The listing builds one solid part. Answer for the finished solid, in the listing's coordinates (mm). A direction names the side the tool comes from. Round coordinates to 2 decimals unless told otherwise and drop trailing zeros. Write each loop counter-clockwise with the first axis right and the second up, starting at its lowest first coordinate (ties: lowest second). Pieces come first, ordered by that corner, then holes. Notation, with made-up numbers: (55.5, -35) -> (79.5, -35) arc R18 ccw to (79.5, -13) -> close; hole circle Ø11 at (56.25, 6.5). An arc over 180 degrees is marked (long way). Write each question's results on one line, items separated by ' | '. Start each with the question number.
Autodesk Inventor part; units mm, degrees
ref_plane "YZ Plane" through (0, 0, 0) normal (1, 0, 0) x (0, 1, 0)
ref_plane "XZ Plane" through (0, 0, 0) normal (0, 1, 0) x (-1, 0, 0)
ref_plane "XY Plane" through (0, 0, 0) normal (0, 0, 1) x (1, 0, 0)
sketch "Sketch1" plane through (0, 0, 0) normal (0, 1, 0) x (-1, 0, 0)
  line L0 (46.6228, 34.6302) -> (-74.0272, 34.6302)
  line L1 (-74.0272, 34.6302) -> (-74.0272, -54.2698)
  line L2 (-74.0272, -54.2698) -> (46.6228, -54.2698)
  line L3 (46.6228, -54.2698) -> (46.6228, 34.6302)
  point P0 (0, 0)
  dimension "d0" = 120.65
  dimension "d1" = 88.9
extrude "Extrusion1" add sketch "Sketch1" along normal blind 12.7
sketch "Sketch2" plane through (0, 12.7, 0) normal (0, 1, 0) x (1, 0, 0)
  line L0 (-46.6228, -34.6302) -> (74.0272, -34.6302)
  line L1 (-46.6228, 54.2698) -> (-46.6228, -34.6302)
  point P0 (0, 0)
  point P1 (6.7172, -29.5502)
  point P2 (51.1672, -29.5502)
  dimension "d4" = 0
  dimension "d5" = 5.08
  dimension "d6" = 53.34
  dimension "d7" = 44.45
hole "Hole1" at (6.7172, 12.7, 29.5502) at (51.1672, 12.7, 29.5502) direction (0, -1, 0) diameter 4.826 depth 25.4 tip angle 118 countersink diameter 9.525 countersink angle 82
sketch "Sketch10" plane through (0, 12.7, 0) normal (0, 1, 0) x (1, 0, 0)
  circle A0 centre (51.1672, -29.5502) radius 2.413
  circle A1 centre (6.7172, -29.5502) radius 2.413
  line L0 (74.0272, 54.2698) -> (-46.6228, 54.2698)
  point P0 (0, 0)
  point P1 (6.7172, 14.2648)
  point P2 (51.1672, 14.2648)
  point P3 (66.6772, 28.8698)
  point P4 (-45.6228, 28.8698)
  point P5 (-46.6228, 54.2698)
  dimension "d80" = 0
  dimension "d81" = 0
  dimension "d82" = 0
  dimension "d144" = 43.815
hole "Hole7" at (6.7172, 12.7, -14.2648) at (51.1672, 12.7, -14.2648) direction (0, -1, 0) diameter 4.826 end through all countersink diameter 9.525 countersink angle 82
sketch "Sketch11" plane through (0, 0, 0) normal (0, -1, 0) x (1, 0, 0)
  line L0 (-28.8428, 29.2002) -> (-16.8428, 29.2002)
  line L1 (-16.8428, 29.2002) -> (-16.8428, 23.2002)
  line L2 (-16.8428, 23.2002) -> (-28.8428, 23.2002)
  line L3 (-28.8428, 23.2002) -> (-28.8428, 29.2002)
  line L4 (-28.8428, -3.8198) -> (-16.8428, -3.8198)
  line L5 (-16.8428, -3.8198) -> (-16.8428, -9.8198)
  line L6 (-16.8428, -9.8198) -> (-28.8428, -9.8198)
  line L7 (-28.8428, -9.8198) -> (-28.8428, -3.8198)
  line L8 (-28.8428, 23.5502) -> (-28.8428, 29.5502)
  line L9 (-16.8428, 29.5502) -> (-16.8428, 23.5502)
  line L10 (74.0272, -54.2698) -> (-46.6228, -54.2698)
  point P0 (0, 0)
  dimension "d93" = 0
  dimension "d94" = 0
  dimension "d95" = 0
  dimension "d96" = 0
  dimension "d97" = 6
  dimension "d98" = 6
  dimension "d99" = 44.45
  dimension "d100" = 77.47
extrude "Extrusion4" cut sketch "Sketch11" against normal blind 1.27
sketch "Sketch13" plane through (0, 0, 0) normal (0, -1, 0) x (1, 0, 0)
  circle A0 centre (-32.8428, -42.0898) radius 1.4
  circle A1 centre (-32.8428, -49.1898) radius 1.4
  line L0 (-46.6228, 34.6302) -> (74.0272, 34.6302)
  circle A2 centre (-11.9428, -42.0898) radius 1.4
  point P0 (0, 0)
  point P1 (-32.8428, -10.3398)
  point P2 (-32.8428, -3.2278)
  point P3 (-32.8428, 22.9462)
  point P4 (-32.8428, 30.0582)
  point P5 (-39.7887, 34.6302)
  point P6 (67.4471, 34.6302)
  point P7 (-11.9428, -10.3398)
  point P8 (-11.9428, -3.2278)
  point P9 (-11.9428, 22.9462)
  point P10 (-11.9428, 30.0582)
  dimension "d110" = 0
  dimension "d111" = 0
  dimension "d112" = 0
  dimension "d113" = 7.112
  dimension "d114" = 7.112
  dimension "d115" = 31.75
  dimension "d116" = 4.572
  dimension "d117" = 0
  dimension "d118" = 0
  dimension "d119" = 0
  dimension "d120" = 0
  dimension "d121" = 0
  dimension "d122" = 0
  dimension "d123" = 0
  dimension "d124" = 0
hole "Hole9" at (-32.8428, 0, -10.3398) at (-32.8428, 0, -3.2278) at (-32.8428, 0, 22.9462) at (-32.8428, 0, 30.0582) at (-11.9428, 0, -10.3398) at (-11.9428, 0, -3.2278) at (-11.9428, 0, 22.9462) at (-11.9428, 0, 30.0582) direction (0, 1, 0) diameter 2.8 end through all
sketch "Sketch15" plane through (0, 12.7, 0) normal (0, 1, 0) x (1, 0, 0)
  circle A0 centre (6.7172, 14.2648) radius 2.413
  circle A1 centre (51.1672, 14.2648) radius 2.413
  circle A2 centre (6.7172, -29.5502) radius 2.413
  circle A3 centre (51.1672, -29.5502) radius 2.413
  circle A4 centre (6.7172, 14.2648) radius 3.3734
  circle A5 centre (6.7172, -29.5502) radius 3.3734
  circle A6 centre (51.1672, -29.5502) radius 3.3734
  circle A7 centre (51.1672, 14.2648) radius 3.3734
  point P0 (0, 0)
  dimension "d138" = 6.7469
  dimension "d139" = 6.7469
  dimension "d140" = 6.7469
  dimension "d141" = 6.7469
extrude "Extrusion6" cut sketch "Sketch15" against normal blind 8.89
sketch "Sketch16" plane through (0, 0, 0) normal (0, -1, 0) x (1, 0, 0)
  line L0 (-64.483, -21.2498) -> (91.0848, -21.2498)
  line L1 (91.0848, -21.2498) -> (91.0848, -72.9236)
  line L2 (91.0848, -72.9236) -> (-64.483, -72.9236)
  line L3 (-64.483, -72.9236) -> (-64.483, -21.2498)
  line L4 (74.0272, -54.2698) -> (-46.6228, -54.2698)
  point P0 (0, 0)
  dimension "d145" = 33.02
extrude "Extrusion7" cut sketch "Sketch16" against normal blind 25.4
sketch "Sketch17" plane through (0, 12.7, 0) normal (0, 1, 0) x (1, 0, 0)
  line L0 (0.9372, 34.8895) -> (84.6395, 34.8895)
  line L1 (84.6395, 34.8895) -> (84.6395, -45.0892)
  line L2 (84.6395, -45.0892) -> (0.9372, -45.0892)
  line L3 (-16.8428, 3.8198) -> (-16.8428, 9.8198)
  line L4 (-46.6228, 21.2498) -> (-46.6228, -34.6302)
  line L5 (-28.8428, 9.8198) -> (-28.8428, 3.8198)
  line L6 (74.0272, 21.2498) -> (-46.6228, 21.2498)
  line L7 (-16.8428, 9.8198) -> (-28.8428, 9.8198)
  line L8 (-60.5333, -6.3402) -> (0.9372, -6.3402)
  line L9 (0.9372, -39.753) -> (-60.5333, -39.753)
  line L10 (-60.5333, -39.753) -> (-60.5333, -6.3402)
  line L11 (0.9372, -45.0892) -> (0.9372, -39.753)
  line L12 (0.9372, -6.3402) -> (0.9372, 34.8895)
  line L13 (-28.8428, 3.8198) -> (-16.8428, 3.8198)
  point P0 (0, 0)
  dimension "d149" = 17.78
  dimension "d150" = 11.43
  dimension "d151" = 10.16
extrude "Extrusion8" cut sketch "Sketch17" against normal blind 25.4 contours L0 L1 L2 L11 L9 L10 L8 L12
sketch "Sketch18" plane through (-46.6228, 0, -21.2498) normal (-1, 0, 0) x (0, 0, 1)
  line L0 (37.4692, 10.16) -> (-18.1099, 10.16)
  line L1 (-18.1099, 10.16) -> (-18.1099, 19.4846)
  line L2 (-18.1099, 19.4846) -> (37.4692, 19.4846)
  line L3 (37.4692, 19.4846) -> (37.4692, 10.16)
  line L4 (0, 12.7) -> (27.59, 12.7)
  point P0 (21.2498, 0)
  dimension "d154" = 2.54
extrude "Extrusion9" cut sketch "Sketch18" against normal blind 55.5625
sketch "Sketch19" plane through (0, 0, 0) normal (0, -1, 0) x (1, 0, 0)
  circle A0 centre (-11.9428, -10.3398) radius 1.4
  circle A1 centre (-32.8428, -10.3398) radius 1.4
  circle A2 centre (-32.8428, -3.2278) radius 1.4
  circle A3 centre (-11.9428, -3.2278) radius 1.4
  line L0 (-28.8428, -9.8198) -> (-28.8428, -3.8198)
  line L1 (-28.8428, -3.8198) -> (-16.8428, -3.8198)
  line L2 (-16.8428, -3.8198) -> (-16.8428, -9.8198)
  line L3 (-16.8428, -9.8198) -> (-28.8428, -9.8198)
  line L4 (0.9372, -21.2498) -> (0.9372, 6.3402)
  line L5 (0.9372, 6.3402) -> (-46.6228, 6.3402)
  line L6 (-46.6228, -21.2498) -> (-46.6228, 6.3402)
  line L7 (-46.6228, -21.2498) -> (0.9372, -21.2498)
  line L8 (0.9372, -21.2498) -> (0.9372, 6.3402)
  line L9 (-46.6228, -21.2498) -> (0.9372, -21.2498)
  line L10 (-46.6228, -21.2498) -> (-46.6228, 6.3402)
  line L11 (-42.8128, 2.5302) -> (-2.8728, 2.5302)
  line L12 (-2.8728, 2.5302) -> (-2.8728, -17.4398)
  line L13 (-2.8728, -17.4398) -> (-42.8128, -17.4398)
  line L14 (-42.8128, -17.4398) -> (-42.8128, 2.5302)
  point P0 (0, 0)
  dimension "d157" = 3.81
  dimension "d158" = 3.81
  dimension "d159" = 3.81
  dimension "d160" = 3.81
extrude "Extrusion10" cut sketch "Sketch19" against normal blind 55.5625 contours L7 L6 L5 L4
equation "\"d125\" = CanConHoleDiam"
equation "\"LegoMainHole\" = 4.8"
equation "\"TalonSRXWidth\" = 31.75"
equation "\"TalonSRXFromSide\" = 15.875"
equation "\"TalonSRXBetweenHoles\" = 50.8"
equation "\"CanConPinWidth\" = 6"
equation "\"CanConPinLength\" = 12"
equation "\"CanConBetweenSideHoles\" = 20.9"
equation "\"CanConBetweenTopHoles\" = 7.1"
equation "\"CanConHoleDiam\" = 2.8"
equation "\"CanConHoleFromTopPin\" = 4"
properties part number "CANConnectorOne"
Q1. Determine the mould class of faces 1 (the flat face through (-23, 1.27, -7)), 2 (the cylindrical face through (-12.363, 5.151, -11.675)), 3 (the flat face through (-23, 10.16, -7)), 4 (the flat face through (-23, 5, -17.44)) for opening direction Z: pulls with the +Z half, pulls with the -Z half, needs draft (parallel to the pull), parting line crosses it, or undercut.
Q2. The part is cut by section B-B, the plane y = 3.75. Write down the section's boundary in (x, z).
Q3. The part is cut by section C-C, the plane z = -3.25. Write down the section's boundary in (x, y).
Q4. The part is cut by section D-D, the plane x = -27.5. Write down the section's boundary in (y, z).
Q5. The part is cut by section A-A, the plane x = -11.5. Write down the section's boundary in (y, z), then the cut area to 3 significant figures.
Q6. Find the intervals of material crossed by line 1 (X direction, y = 5.25, z = -3.25); line 2 (Z direction, x = -12, y = 7.5); line 3 (X direction, y = 1, z = -5.5), in increasing order.
Q7. For faces 5 (the cylindrical face through (-34.23, 5.15, -3.05)), 6 (the flat face through (-28.843, 1, -7)), determine the directions among +Z, -Z, +X, -X, +Y, -Y from which every point of the face is accessible in a straight line to the end or side of a thin tool.
Answers follow:
1) face 1: undercut | face 2: undercut | face 3: needs draft | face 4: pulls with the -Z half
2) outline: (-42.81, -17.44) -> (-2.87, -17.44) -> (-2.87, 2.53) -> (-42.81, 2.53) -> close; hole circle Ø2.8 at (-32.84, -10.34); hole circle Ø2.8 at (-32.84, -3.23); hole circle Ø2.8 at (-11.94, -10.34); hole circle Ø2.8 at (-11.94, -3.23)
3) outline: (-42.81, 0) -> (-34.24, 0) -> (-34.24, 10.16) -> (-42.81, 10.16) -> close; (-31.44, 0) -> (-13.34, 0) -> (-13.34, 10.16) -> (-31.44, 10.16) -> close; (-10.54, 0) -> (-2.87, 0) -> (-2.87, 10.16) -> (-10.54, 10.16) -> close
4) outline: (0, -17.44) -> (10.16, -17.44) -> (10.16, 2.53) -> (0, 2.53) -> (0, -3.82) -> (1.27, -3.82) -> (1.27, -9.82) -> (0, -9.82) -> close
5) outline: (0, -17.44) -> (10.16, -17.44) -> (10.16, -11.67) -> (0, -11.67) -> close; (0, -9.01) -> (10.16, -9.01) -> (10.16, -4.56) -> (0, -4.56) -> close; (0, -1.9) -> (10.16, -1.9) -> (10.16, 2.53) -> (0, 2.53) -> close | area: 149 mm^2
6) line 1: -42.81 to -34.24, -31.44 to -13.34, -10.54 to -2.87 | line 2: -17.44 to -11.74, -8.94 to -4.63, -1.83 to 2.53 | line 3: -42.81 to -28.84, -16.84 to -2.87
7) face 5: +Y, -Y | face 6: -Y
